Source: CAD feature listing. Evaluate the final solid. Frame: model axes, mm. Face numbers are marked on the shaded views. A direction names the side the tool comes from. Coordinates: 2 decimals unless noted, no trailing zeros. Write each loop counter-clockwise with the first axis right and the second up, starting at its lowest first coordinate (ties: lowest second). Pieces come first, ordered by that corner, then holes. Notation, with made-up numbers: (-22.5, 71.25) - (35.5, 71.25) arc R12 ccw to (35.5, 89.25) - close; hole circle Ø1 at (18.25, 87). An arc over 180 degrees is marked (long way). One line per question, with ' | ' between items. Start each with the question number.
Q1. Cut plane D-D, the plane z = 30.5. Return loops of the section in (x, y).
Q2. Cut plane B-B, the plane y = -1. Return loops of the section in (x, z) (3 decimals), plus the area to 3 significant figures.
Q3. Draft query along Y for the marked faces 6, 7 and 8. Return one class per face: +Y half, -Y half, draft (parallel to the pull), parting line (faces both ways), or undercut.
Q4. Access query for the marked faces 1, 2, 3, 4 and 5. Directions: +Z, -Z, +X, -X, +Y, -Y. A direction counts if a zero-diameter tool reaches every point of the face in a straight line with its end or side. Return the directions, or none.
Q5. Line query: line 1 (X direction, y = -12.5, z = -4); line 2 (X direction, y = 1, z = 13). Output: solid intervals per line, ascending.
Q6. Contact query for flat-ended pins moving along their axis: P1, Ø24.5, axis at x = 25, z = -3, coming from the -Y side; P2, Ø6.5, axis at y = 28, z = -5.5, coming from the -X side; P3, Ø6.5, axis at x = -2, y = 27, coming from the -Z side. Output: stop coordinate, or through.
Q7. Cut plane A-A, the plane z = -1.5. Return loops of the section in (x, y) (3 decimals).
Q8. Cut plane C-C, the plane x = 0. Return loops of the section in (y, z) (3 decimals), plus the area to 3 significant figures.
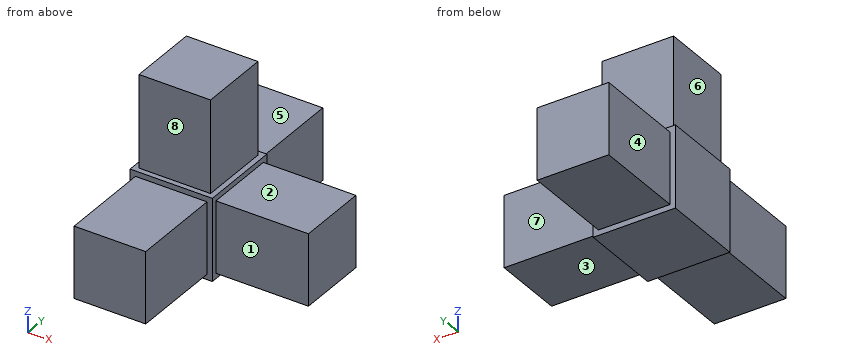
```python
from build123d import *

# Parameters (mm, degrees)
F0_W     = 22.098
F0_H     = 22.098
F1_DEPTH = 41.275
F2_DEPTH = 12.7
F0_H_2   = 28.575
F3_DEPTH = 11.049
F0_W_2   = 28.575
F4_DEPTH = 11.049


with BuildPart() as f1:
    # F0 (on Front) → F1 (new body, symmetric)
    with BuildSketch(Plane.XZ):
        Rectangle(F0_W, F0_H)
    extrude(amount=F1_DEPTH, both=True)

    # F0 (on Front) → F2 (join, symmetric)
    with BuildSketch(Plane.XZ):
        Polygon((-11.049, 12.7), (-12.7, 12.7), (-12.7, -12.7), (12.7, -12.7), (12.7, -11.049), (12.7, 11.049), (12.7, 12.7), (11.049, 12.7), align=None)
        Rectangle(F0_W, F0_H, mode=Mode.SUBTRACT)
        Rectangle(F0_W, F0_H)
    extrude(amount=F2_DEPTH, both=True)

    # F0 (on Front) → F3 (join, symmetric)
    with BuildSketch(Plane.XZ):
        with Locations((0, 26.9875)):
            Rectangle(F0_W, F0_H_2)
    extrude(amount=F3_DEPTH, both=True)

    # F0 (on Front) → F4 (join, symmetric)
    with BuildSketch(Plane.XZ):
        with Locations((26.9875, 0)):
            Rectangle(F0_W_2, F0_H)
    extrude(amount=F4_DEPTH, both=True)


solid = f1.part
```
Reply:
1) outline: (-11.05, -11.05) - (11.05, -11.05) - (11.05, 11.05) - (-11.05, 11.05) - close
2) outline: (-12.7, -12.7) - (12.7, -12.7) - (12.7, -11.049) - (41.275, -11.049) - (41.275, 11.049) - (12.7, 11.049) - (12.7, 12.7) - (11.049, 12.7) - (11.049, 41.275) - (-11.049, 41.275) - (-11.049, 12.7) - (-12.7, 12.7) - close | area: 1,910 mm^2
3) face 6: draft | face 7: +Y half | face 8: -Y half
4) face 1: +Z, -Z, +X, -Y | face 2: +Z, +X, +Y, -Y | face 3: -Z, +X, +Y, -Y | face 4: +Z, -Z, -X, +Y | face 5: +Z, +X, -X, +Y
5) line 1: x = -12.7 to 12.7 | line 2: x = -11.05 to 11.05
6) P1: stops at y = -11.05 | P2: stops at x = -11.05 | P3: stops at z = -11.05
7) outline: (-12.7, -12.7) - (-11.049, -12.7) - (-11.049, -41.275) - (11.049, -41.275) - (11.049, -12.7) - (12.7, -12.7) - (12.7, -11.049) - (41.275, -11.049) - (41.275, 11.049) - (12.7, 11.049) - (12.7, 12.7) - (11.049, 12.7) - (11.049, 41.275) - (-11.049, 41.275) - (-11.049, 12.7) - (-12.7, 12.7) - close
8) outline: (-41.275, -11.049) - (-12.7, -11.049) - (-12.7, -12.7) - (12.7, -12.7) - (12.7, -11.049) - (41.275, -11.049) - (41.275, 11.049) - (12.7, 11.049) - (12.7, 12.7) - (11.049, 12.7) - (11.049, 41.275) - (-11.049, 41.275) - (-11.049, 12.7) - (-12.7, 12.7) - (-12.7, 11.049) - (-41.275, 11.049) - close | area: 2,540 mm^2
